The model under review builds one solid part; all positions refer to its coordinate system, in mm. Face numbers are marked on the shaded views. A direction names the side the tool comes from. Give positions to 0.01 mm unless a question says otherwise; leave off trailing zeros. Order: outer loops, then holes, each group sorted by start corner. A loop starts at its lowest first (then second) coordinate and runs counter-clockwise, first axis right, second up.
```python
from build123d import *

# Parameters (mm, degrees)
F8_W     = 203.2
F8_H     = 101.6
F0_DEPTH = 25.4
F1_W     = 203.2
F1_H     = 25.4
F2_DEPTH = 101.6
F9_DEPTH = 25.4
F4_R     = 25.4
F5_R     = 50.8
F6_DEPTH = 25.4
F7_DEPTH = 25.4


with BuildPart() as f0:
    # F8 (on Top) → F0 (new body)
    with BuildSketch(Plane.XY):
        with Locations((55.668721, -12.031432)):
            Rectangle(F8_W, F8_H)
    extrude(amount=F0_DEPTH)

    # F1 (on face) → F2 (join)
    with BuildSketch(Plane.XY.offset(25.4)):
        with Locations((55.668721, 26.068568)):
            Rectangle(F1_W, F1_H)
    extrude(amount=F2_DEPTH)

    # F3 (on face) → F9 (cut)
    with BuildSketch(Plane.XZ.offset(-13.368568)):
        with BuildLine():
            Line((157.268721, 101.6), (157.268721, 127))
            Line((157.268721, 127), (131.868721, 127))
            ThreePointArc((131.868721, 127), (149.829233, 119.560512), (157.268721, 101.6))
        make_face()
    extrude(amount=-F9_DEPTH, mode=Mode.SUBTRACT)

    # F4
    f4_edges = [f0.edges().sort_by_distance(p)[0] for p in [
        (-45.931279, 26.068568, 127),
    ]]
    fillet(f4_edges, radius=F4_R)

    # F5 (on face) → F6 (cut)
    with BuildSketch(Plane.XY.offset(25.4)):
        with Locations((47.562543, -62.831432)):
            Circle(F5_R)
    extrude(amount=-F6_DEPTH, mode=Mode.SUBTRACT)

    # F0_face (on face) → F7 (join)
    with BuildSketch(Plane(origin=(55.668721, -12.031432, 25.4), x_dir=(1, 0, 0), z_dir=(0, 0, 1))):
        with BuildLine():
            Line((42.693822, -50.8), (101.6, -50.8))
            Line((101.6, -50.8), (101.6, 25.4))
            Line((101.6, 25.4), (-101.6, 25.4))
            Line((-101.6, 25.4), (-101.6, -50.8))
            Line((-101.6, -50.8), (-58.906178, -50.8))
            ThreePointArc((-58.906178, -50.8), (-8.106178, 0), (42.693822, -50.8))
        make_face()
    extrude(amount=F7_DEPTH)


solid = f0.part
```
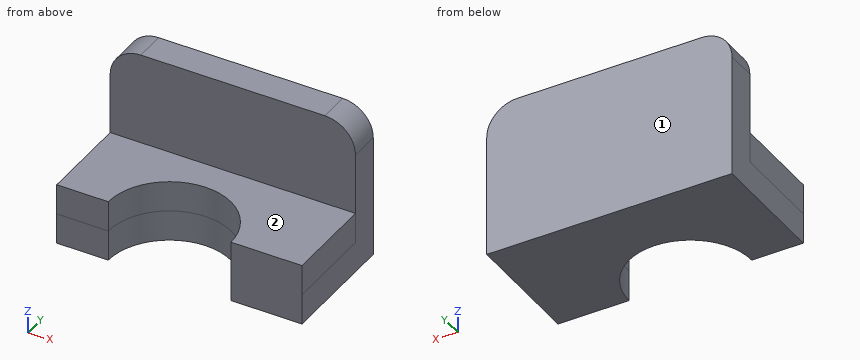
1. Insertion check: pin 1 (2 mm diameter, centred on x = 133, y = -19, fed in from +Z); pin 2 (23 mm diameter, centred on x = 74, z = 74.5, fed in from -Y). Each pin has a flat end and moves straight along its axis. Give the tip position at first contact, or say it passes through.
2. Take a section at C-C (x = 116.5). Write out the cut boundary in (y, z).
3. Take a section at A-A (y = -23). Write out the cut boundary in (x, z).
4. For the marked faces 1 and 2, list the 3-axis set-ups (+Z, -Z, +X, -X, +Y, -Y) from which the entire face can be reached by the end or side of a thin tool; tool diameter is ignored.
5. Take a section at B-B (z = 11). Write out the cut boundary in (x, y), and give its area (3 significant figures).
6. Take a section at D-D (y = -46.5). Write out the cut boundary in (x, z), and give its area (3 significant figures).
7. To check wall thickness, follow line 1 (Z direction, x = -10, y = -50); line 2 (Y direction, x = 0, z = 110); line 3 (X direction, y = -31, z = 49). State the ranges of each line that lie inside material, in increasing order.
Answer:
1. pin 1: stops at z = 50.8
1. pin 2: stops at y = 13.37
2. outline: (-62.83, 0) - (38.77, 0) - (38.77, 127) - (13.37, 127) - (13.37, 50.8) - (-62.83, 50.8) - close
3. outline: (-45.93, 0) - (16.03, 0) - (16.03, 50.8) - (-45.93, 50.8) - close; (79.09, 0) - (157.27, 0) - (157.27, 50.8) - (79.09, 50.8) - close
4. face 1: +Z, -Z, +X, -X, +Y
4. face 2: +Z, +X, -X, -Y
5. outline: (-45.93, -62.83) - (-3.24, -62.83) arc R50.8 cw to (98.36, -62.83) - (157.27, -62.83) - (157.27, 38.77) - (-45.93, 38.77) - close
5. area: 16,600 mm2
6. outline: (-45.93, 0) - (-0.54, 0) - (-0.54, 50.8) - (-45.93, 50.8) - close; (95.67, 0) - (157.27, 0) - (157.27, 50.8) - (95.67, 50.8) - close
6. area: 5,440 mm2
7. line 1: z = 0 to 50.8
7. line 2: y = 13.37 to 38.77
7. line 3: x = -45.93 to 7.97, 87.15 to 157.27
